Geometry check sheet. Reference: the model listing, model coordinates, mm. A direction names the side the tool comes from. Coordinates: 2 decimals unless noted, no trailing zeros. Put each result on its own line as item: value. Start each with the question number.
1) Gauge pin test, flat ends, axial feed: pin 1 (1.5 mm diameter, centred on x = -1, y = 2, fed in from -Z); pin 2 (1.8 mm diameter, centred on x = 0.5, z = -1, fed in from -Y); pin 3 (2 mm diameter, centred on y = 5, z = 0, fed in from -X). Record the tip position at first contact, or that the pin passes through.
2) Scan lines: line 1 along X through (y, z) = (5.8, 0); line 2 along Z through (x, y) = (-0.25, 6.5); line 3 along X through (y, z) = (6.05, 0). Record each from-to range of solid material in increasing order.
3) Mould release check, pull along X, two halves, no side actions. Record for faces 1 (the flat face through (-2.2, 0, -2.3)), 2 (the flat face through (0.502, 1.085, -2.704)), 3 (the flat face through (2.6, 1.1, -0.9)): released by +X, released by -X, zero draft, split by the parting line, or undercut.
4) Set-up check for faces 4 (the flat face through (-1.4, 2.2, 1.4)), 5 (the cylindrical face through (-1.5, 4.61, 0.07)): record each of +Z, -Z, +X, -X, +Y, -Y from which the full face is reachable in a straight line by a thin tool's end or side.
from build123d import *

# Parameters (mm, degrees)
F2_R     = 1.5
F3_DEPTH = 25
F4_DEPTH = 2.2


with BuildPart() as f1:
    # F0 (on Top) → F1 (revolve)
    with BuildSketch(Plane.XY):
        with BuildLine():
            Line((0, 8.115384), (0, 0))
            Line((0, 0), (5, 0))
            ThreePointArc((5, 0), (3.571673, 4.717964), (0, 8.115384))
        make_face()
    revolve(axis=Axis((0, 4.057692, 0), (0, 1, 0)))

    # F2 (on face) → F3 (cut)
    with BuildSketch(Plane.XZ):
        Circle(F2_R)
    extrude(amount=-F3_DEPTH, mode=Mode.SUBTRACT)

    # F2 (on face) → F4 (cut)
    with BuildSketch(Plane.XZ):
        Polygon((3.117215, 0.605232), (1.034461, 3.002203), (-2.082754, 2.396971), (-3.117215, -0.605232), (-1.034461, -3.002203), (2.082754, -2.396971), align=None)
        Circle(F2_R, mode=Mode.SUBTRACT)
    extrude(amount=-F4_DEPTH, mode=Mode.SUBTRACT)


solid = f1.part
Answer key:
1. pin 1: stops at z = -4.82
1. pin 2: stops at y = 2.2
1. pin 3: stops at x = -3.97
2. line 1: x = -2.8 to -1.5, 1.5 to 2.8
2. line 2: z = -2.14 to -1.48, 1.48 to 2.14
2. line 3: x = -2.58 to -1.5, 1.5 to 2.58
3. face 1: zero draft
3. face 2: undercut
3. face 3: undercut
4. face 4: -Y
4. face 5: +Y, -Y
